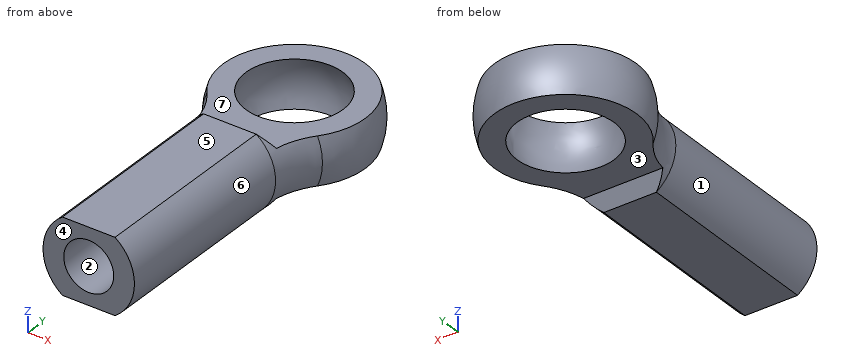
from build123d import *

# Parameters (mm, degrees)
SKETCH17_W              = 7.1501
SKETCH17_H              = 68.2625
EXTRUDE3_DEPTH          = 63.5
CUT_EXTRUDE1_DEPTH      = 45.878768644
CUT_EXTRUDE1_DEPTH_BACK = 45.878768644


with BuildPart() as part:
    # Sketch15 → Revolve4 (revolve)
    with BuildSketch(Plane.XY, mode=Mode.PRIVATE) as revolve4_sk:
        Polygon((4.7625, -26.9875), (8.7249, -26.9875), (8.7249, 10.047604155), (0, 10.047604155), (0, 0), (4.7625, 0), align=None)
    revolve(revolve4_sk.sketch.rotate(Axis((0, 41.275, 0), (0, -1, 0)), 180), axis=Axis((0, 41.275, 0), (0, -1, 0)))

    # Sketch4 → Revolve2 (revolve)
    with BuildSketch(Plane.XY):
        with BuildLine():
            Line((0, 16.6751), (0, 10.047604155))
            Line((0, 10.047604155), (8.7249, 10.047604155))
            ThreePointArc((8.7249, 10.047604155), (9.438021768, 14.505059918), (11.5062, 18.517552077))
            ThreePointArc((11.5062, 18.517552077), (12.750432094, 33.434137701), (0, 41.275))
            Line((0, 41.275), (0, 37.2999))
            ThreePointArc((0, 37.2999), (10.3124, 26.9875), (0, 16.6751))
        make_face()
    revolve(axis=Axis((0, 41.275, 0), (0, 1, 0)))

    # Sketch17 → Extrude3 (cut, symmetric)
    with BuildSketch(Plane(origin=(0, 0, 0), x_dir=(0, 0, -1), z_dir=(1, 0, 0))):
        with Locations((-10.71245, 7.14375)):
            Rectangle(SKETCH17_W, SKETCH17_H)
        with Locations((10.71245, 7.14375)):
            Rectangle(SKETCH17_W, SKETCH17_H)
    extrude(amount=EXTRUDE3_DEPTH, both=True, mode=Mode.SUBTRACT)

    # Sketch5 → Cut-Extrude1 (cut, two sides: drawn at the far end of the back side and taken through both)
    with BuildSketch(Plane(origin=(0, 0, 0), x_dir=(0, 0, -1), z_dir=(1, 0, 0)).offset(-CUT_EXTRUDE1_DEPTH_BACK)):
        Polygon((4.5640625, 41.275), (12.2174, 41.275), (12.2174, 10.047604155), (7.1374, 10.047604155), (4.5640625, 11.873229155), align=None)
        Polygon((-4.5640625, 41.275), (-4.5640625, 11.873229155), (-7.1374, 10.047604155), (-12.2174, 10.047604155), (-12.2174, 41.275), align=None)
    extrude(amount=CUT_EXTRUDE1_DEPTH + CUT_EXTRUDE1_DEPTH_BACK, mode=Mode.SUBTRACT)


solid = part.part
Input: part model. Units: mm. Frame: model coordinates. Face numbers are marked on the shaded views. A direction names the side the tool comes from. Round coordinates to 2 decimals unless told otherwise and drop trailing zeros. Loops run counter-clockwise (first coordinate to the right, second up) from the corner with the lowest first, then second, coordinate; pieces in that order, holes last. Notation, with made-up numbers: (85.25, 22) -> (97.25, 22) arc R30 cw to (97.25, 59) -> close; hole circle Ø1 at (76.5, 85.25). An arc over 180 degrees is marked (long way). Answer as a JSON object with one key per item and string values. Group by question number.
1) Section query D-D on y = 7. Output: boundary loops of the cut face in (x, z).
2) Ray query, L1, parallel to Z at x = 0, y = -12.5; L2, parallel to X at y = -24, z = 0.25; L3, parallel to Y at x = -4, z = 0. Return the intervals inside material, ascending.
3) Section query A-A on z = 0. Output: boundary loops of the cut face in (x, y) (1 decimal).
4) Pin query (flat end, axial travel): pin 1 (4 mm diameter, centred on x = 3, y = 31.5, fed in from -Z) (3 decimals); pin 2 (5 mm diameter, centred on y = -14.5, z = 3, fed in from -X); pin 3 (2 mm diameter, centred on x = -8.5, z = 3, fed in from +Y); pin 4 (8 mm diameter, centred on x = -4, y = -16.5, fed in from +Z). Return the tip coordinate at first contact, or that it passes through.
5) Section query B-B on x = 0. Output: boundary loops of the cut face in (y, z) (1 decimal).
6) Draft query along Z for the marked faces 1, 2, 3 and 4. Return one class per face: +Z half, -Z half, draft (parallel to the pull), parting line (faces both ways), or undercut.
7) Section query C-C on y = 34. Output: boundary loops of the cut face in (x, z).
8) Reachability of the marked faces 5, 6 and 7 from +Z, -Z, +X, -X, +Y, -Y: full face, straight path, thin tool, end or side. Return the list, or none.
Reply:
{
 "1": {"outline": "(-5.02, -7.14) -> (5.02, -7.14) arc R8.72 ccw to (5.02, 7.14) -> (-5.02, 7.14) arc R8.72 ccw to start"},
 "2": {"L1": "z = -7.14 to -4.76, 4.76 to 7.14", "L2": "x = -8.72 to -4.76, 4.76 to 8.72", "L3": "y = 0 to 17.48, 36.49 to 40.7"},
 "3": {"outline": "(-11.5, 18.5) arc R14.3 cw to (-8.7, 10) -> (-8.7, -27) -> (-4.8, -27) -> (-4.8, 0) -> (4.8, 0) -> (4.8, -27) -> (8.7, -27) -> (8.7, 10) arc R14.3 cw to (11.5, 18.5) arc R14.3 ccw (long way) to start; hole circle Ø20.6 at (0, 27)"},
 "4": {"pin 1": "passes through", "pin 2": "stops at x = -8.71", "pin 3": "stops at y = 38.82", "pin 4": "stops at z = 7.14"},
 "5": {"outline": "(-27, -7.1) -> (10, -7.1) -> (11.9, -4.6) -> (17.7, -4.6) arc R10.3 cw to (17.7, 4.6) -> (11.9, 4.6) -> (10, 7.1) -> (-27, 7.1) -> (-27, 4.8) -> (0, 4.8) -> (0, -4.8) -> (-27, -4.8) -> close; (36.2, -4.6) -> (40.5, -4.6) arc R14.3 ccw to (40.5, 4.6) -> (36.2, 4.6) arc R10.3 cw to start"},
 "6": {"face 1": "parting line", "face 2": "undercut", "face 3": "-Z half", "face 4": "draft"},
 "7": {"outline": "(-11.58, -4.56) -> (-6.03, -4.56) arc R7.56 cw to (-6.03, 4.56) -> (-11.58, 4.56) arc R12.45 ccw to start; (6.03, -4.56) -> (11.58, -4.56) arc R12.45 ccw to (11.58, 4.56) -> (6.03, 4.56) arc R7.56 cw to start"},
 "8": {"face 5": "+Z, +X, -X, +Y, -Y", "face 6": "+X, -Y", "face 7": "+Z, +X, -X, +Y"}
}
